Geometry: see drawing. Coordinates: mm, zero at the bounding-box minimum. A direction names the side the tool comes from. Give positions to 0.01 mm unless a question says otherwise; leave off trailing zeros. Loops run counter-clockwise (first coordinate to the right, second up) from the corner with the lowest first, then second, coordinate; pieces in that order, holes last. Notation, with made-up numbers: (65, -29.5) - (120, -29.5) arc R19 cw to (120, 6.5) - close; hole circle Ø8 at (61, -5.75). An arc over 180 degrees is marked (long way). Use one line per item in the form item = value.
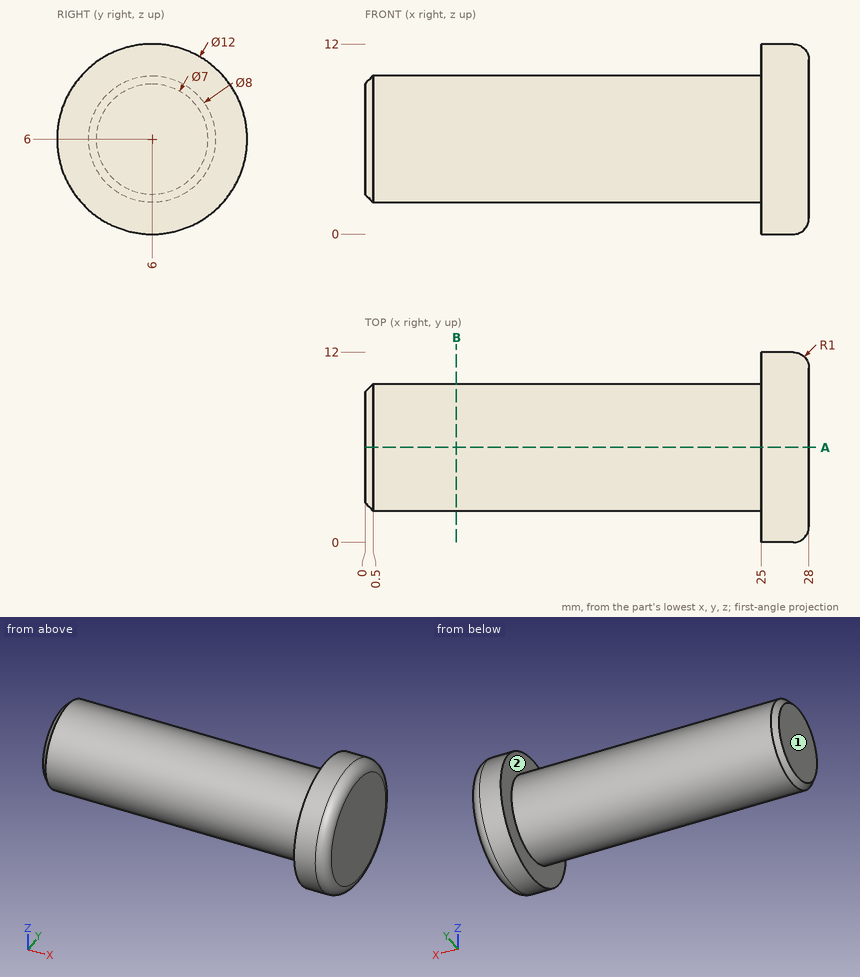
(1) Access query for the marked faces 1 and 2. Directions: +Z, -Z, +X, -X, +Y, -Y. A direction counts if a zero-diameter tool reaches every point of the face in a straight line with its end or side. Return the directions, or none.
Solution:
face_1 = +Z, -Z, -X, +Y, -Y
face_2 = -X
(2) Cut plane A-A (y = 6). Return the cut outline in (x, z), plus the area to 3 significant figures.
Solution:
outline = (0, 2.5) - (0.5, 2) - (25, 2) - (25, 0) - (27, 0) arc R1 ccw to (28, 1) - (28, 11) arc R1 ccw to (27, 12) - (25, 12) - (25, 10) - (0.5, 10) - (0, 9.5) - close
area = 235 mm2
(3) Pin query (flat end, axial travel): P1, Ø1, axis at x = 22, y = 2.5, coming from the +Z side; P2, Ø1.5, axis at y = 7.5, z = 3.5, coming from the -X side; P3, Ø3, axis at x = 18.5, z = 2.5, coming from the -Y side. Return the tip coordinate at first contact, or that it passes through.
Solution:
P1 = 8.65
P2 = 0
P3 = 2.54
(4) Material intervals for L1, parallel to Y at x = 13.5, z = 6; L2, parallel to X at y = 7.5, z = 10.25; L3, parallel to Z at x = 8.5, y = 3.25, sorted ascending. Write a range as from..to.
Solution:
L1 = 2..10
L2 = 25..28
L3 = 3.1..8.9
(5) Cut plane B-B (x = 5.75). Return the cut outline in (y, z), plus the area to 3 significant figures.
Solution:
outline = circle Ø8 at (6, 6)
area = 50.3 mm2
